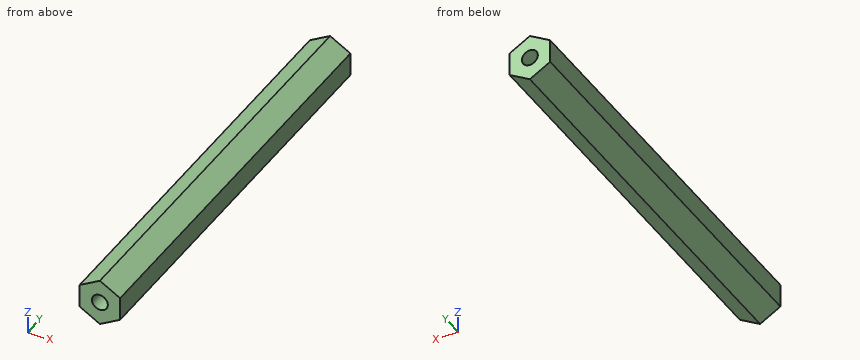
Autodesk Inventor part; units mm, degrees
ref_plane "YZ Plane" through (0, 0, 0) normal (1, 0, 0) x (0, 1, 0)
ref_plane "XZ Plane" through (0, 0, 0) normal (0, 1, 0) x (-1, 0, 0)
ref_plane "XY Plane" through (0, 0, 0) normal (0, 0, 1) x (1, 0, 0)
sketch "Sketch1" plane through (0, 0, 0) normal (0, 1, 0) x (-1, 0, 0)
  line L0 (6.35, -3.6662) -> (0, -7.3323)
  line L1 (0, -7.3323) -> (-6.35, -3.6662)
  line L2 (-6.35, -3.6662) -> (-6.35, 3.6662)
  line L3 (-6.35, 3.6662) -> (0, 7.3323)
  line L4 (0, 7.3323) -> (6.35, 3.6662)
  line L5 (6.35, 3.6662) -> (6.35, -3.6662)
  point P0 (0, 0)
  point P1 (0, 0)
  point P2 (0, 0)
  dimension "d0" = 12.7
extrude "Extrusion1" add sketch "Sketch1" along normal blind 130.1242
sketch "Sketch2" plane through (0, 0, 0) normal (0, -1, 0) x (1, 0, 0)
  point P0 (0, 0)
  point P1 (0, 0)
hole "Hole1" at (0, 0, 0) direction (0, 1, 0) diameter 4.9784 depth 25.4
sketch "Sketch3" plane through (0, 130.1242, 0) normal (0, 1, 0) x (1, 0, 0)
  point P0 (0, 0)
  point P1 (0, 0)
hole "Hole2" at (0, 130.1242, 0) direction (0, -1, 0) diameter 4.9784 depth 25.4
properties part number "SHOT_1_006_HexShaft1" material "Aluminum 6061"
Work out the finished part from the listing and answer in its coordinate system (mm). Round coordinates to 2 decimals unless told otherwise and drop trailing zeros. Write each loop counter-clockwise with the first axis right and the second up, starting at its lowest first coordinate (ties: lowest second). Pieces come first, ordered by that corner, then holes. Notation, with made-up numbers: (78, 26.25) -> (124, 26.25) arc R30 cw to (124, 56.25) -> close; hole circle Ø1 at (63.5, 46.5). An arc over 180 degrees is marked (long way). Answer as CSV lines item,"result". Start each with the question number.
(1) The part is cut by section D-D, the plane z = 5.25. Give the vertices of the cut face in (x, y), then the cut area to 3 significant figures.
(2) Find the intervals of material crossed by probe 1 along X at (y, z) = (119.25, 0); probe 2 along Z at (x, y) = (0, 116.5); probe 3 along X at (y, z) = (11.5, 1.5), in increasing order.
(3) Each of these flat-tipped pins is pushed along its axis until it touches: pin 1 (6 mm diameter, centred on x = 0, y = 58, fed in from +Z); pin 2 (3 mm diameter, centred on x = 0, z = 0, fed in from -Y); pin 3 (5 mm diameter, centred on x = -4.5, y = 88, fed in from +Z). Where does it stop, or does it pass through?
(4) The part is cut by section B-B, the plane y = 50.5. Give the vertices of the cut face in (x, z).
(5) The part is cut by section A-A, the plane z = 0. Give the vertices of the cut face in (x, y).
(6) The part is cut by section C-C, the plane x = 4. Give the vertices of the cut face in (y, z).
Output values:
1,outline,"(-3.61, 0) -> (3.61, 0) -> (3.61, 130.12) -> (-3.61, 130.12) -> close"
1,area,"939 mm²"
2,probe 1,"x = -6.35 to -2.49, 2.49 to 6.35"
2,probe 2,"z = -7.33 to -2.49, 2.49 to 7.33"
2,probe 3,"x = -6.35 to -1.99, 1.99 to 6.35"
3,pin 1,"stops at z = 7.33"
3,pin 2,"stops at y = 25.4"
3,pin 3,"stops at z = 6.18"
4,outline,"(-6.35, -3.67) -> (0, -7.33) -> (6.35, -3.67) -> (6.35, 3.67) -> (0, 7.33) -> (-6.35, 3.67) -> close"
5,outline,"(-6.35, 0) -> (-2.49, 0) -> (-2.49, 25.4) -> (2.49, 25.4) -> (2.49, 0) -> (6.35, 0) -> (6.35, 130.12) -> (2.49, 130.12) -> (2.49, 104.72) -> (-2.49, 104.72) -> (-2.49, 130.12) -> (-6.35, 130.12) -> close"
6,outline,"(0, -5.02) -> (130.12, -5.02) -> (130.12, 5.02) -> (0, 5.02) -> close"
